```python
from build123d import *

# Parameters (mm, degrees)
ESQUISSE3_W             = 50
ESQUISSE3_H             = 100
BOSS_EXTRU_2_DEPTH      = 10
CONG_1_R                = 15
ESQUISSE4_R             = 5
ESQUISSE4_R_2           = 7.5
ENL_V_MAT_EXTRU_1_DEPTH = 10


with BuildPart() as part:
    # Esquisse3 → Boss.-Extru.2 (new body)
    with BuildSketch(Plane.XY):
        Rectangle(ESQUISSE3_W, ESQUISSE3_H)
    extrude(amount=BOSS_EXTRU_2_DEPTH)

    # Congé1
    cong_1_edges = [part.edges().sort_by_distance(p)[0] for p in [
        (-25, 50, 5),
        (25, 50, 5),
        (25, -50, 5),
        (-25, -50, 5),
    ]]
    fillet(cong_1_edges, radius=CONG_1_R)

    # Esquisse4 → Enlèv. mat.-Extru.1 (cut)
    with BuildSketch(Plane(origin=(0, 0, 0), x_dir=(-1, 0, 0), z_dir=(0, 0, -1))):
        with Locations((0, -25)):
            Circle(ESQUISSE4_R)
        with Locations((0, 25)):
            Circle(ESQUISSE4_R)
        Circle(ESQUISSE4_R_2)
    extrude(amount=-ENL_V_MAT_EXTRU_1_DEPTH, mode=Mode.SUBTRACT)


solid = part.part
```
The listing builds one solid part. Answer for the finished solid, in the listing's coordinates (mm). Give positions to 0.01 mm unless a question says otherwise; leave off trailing zeros. Write each loop counter-clockwise with the first axis right and the second up, starting at its lowest first coordinate (ties: lowest second). Pieces come first, ordered by that corner, then holes. Notation, with made-up numbers: (23, 84.25) -> (56, 84.25) arc R30 ccw to (56, 114.25) -> close; hole circle Ø3 at (55, 12.5). An arc over 180 degrees is marked (long way). Use one line per item in the form item = value.
1) Section A-A on y = 25 is taken. Write down the section's boundary in (x, z), plus the area to 3 significant figures.
Result:
outline = (-25, 0) -> (-5, 0) -> (-5, 10) -> (-25, 10) -> close; (5, 0) -> (25, 0) -> (25, 10) -> (5, 10) -> close
area = 400 mm²
2) Each of these flat-tipped pins is pushed along its axis until it touches: P1, Ø3, axis at x = 8, y = -5, coming from the -Z side; P2, Ø9, axis at x = 0, y = 0, coming from the -Z side. Where does it stop, or does it pass through?
Result:
P1 = 0
P2 = through
3) Section C-C on z = 1 is taken. Write down the section's boundary in (x, y), plus the area to 3 significant figures.
Result:
outline = (-25, -35) arc R15 ccw to (-10, -50) -> (10, -50) arc R15 ccw to (25, -35) -> (25, 35) arc R15 ccw to (10, 50) -> (-10, 50) arc R15 ccw to (-25, 35) -> close; hole circle Ø15 at (0, 0); hole circle Ø10 at (0, -25); hole circle Ø10 at (0, 25)
area = 4,470 mm²
4) For a pull along Y with two mould halves and no side action, classify faces 1 (the cylindrical face through (1.08, -29.88, 4.93)), 2 (the flat face through (0, -50, 5)), 3 (the flat face through (25, 0, 5)) as +Y half, -Y half, draft (parallel to the pull), parting line (faces both ways), or undercut.
Result:
face_1 = undercut
face_2 = -Y half
face_3 = draft
5) Section D-D on y = 0 is taken. Write down the section's boundary in (x, z), plus the area to 3 significant figures.
Result:
outline = (-25, 0) -> (-7.5, 0) -> (-7.5, 10) -> (-25, 10) -> close; (7.5, 0) -> (25, 0) -> (25, 10) -> (7.5, 10) -> close
area = 350 mm²
6) Section B-B on x = 0 is taken. Write down the section's boundary in (y, z).
Result:
outline = (-50, 0) -> (-30, 0) -> (-30, 10) -> (-50, 10) -> close; (-20, 0) -> (-7.5, 0) -> (-7.5, 10) -> (-20, 10) -> close; (7.5, 0) -> (20, 0) -> (20, 10) -> (7.5, 10) -> close; (30, 0) -> (50, 0) -> (50, 10) -> (30, 10) -> close
7) Straight lines are drawn through the part: probe 1 along Y at (x, z) = (0, 3.75); probe 2 along Y at (x, z) = (-12, 3.75); probe 3 along X at (y, z) = (-2, 1.5). For each, find the intervals that lie inside material, in ascending order.
Result:
probe_1 = -50 to -30, -20 to -7.5, 7.5 to 20, 30 to 50
probe_2 = -49.87 to 49.87
probe_3 = -25 to -7.23, 7.23 to 25
